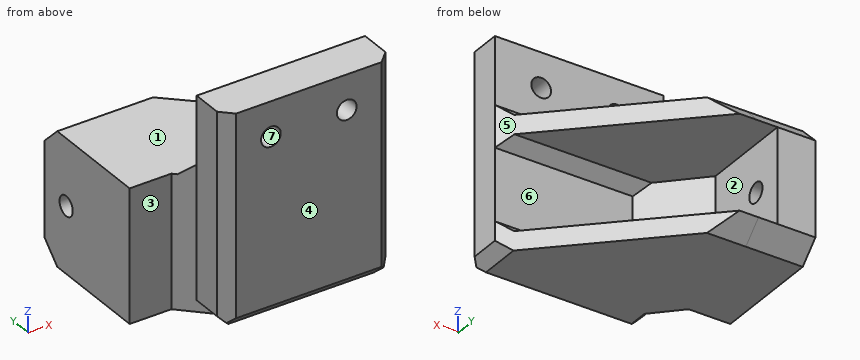
```python
from build123d import *

# Parameters (mm, degrees)
SKETCH2_W                = 44.4
SKETCH2_H                = 55.82
BOSS_EXTRUDE1_DEPTH      = 11
CHAMFER1_SIZE            = 3
SKETCH3_R                = 2.6
CUT_EXTRUDE1_DEPTH       = 62.071371362
SKETCH4_W                = 35
SKETCH4_H                = 37.5
SKETCH4_R                = 2.6
BOSS_EXTRUDE2_DEPTH      = 5
BOSS_EXTRUDE7_DEPTH      = 5
BOSS_EXTRUDE9_DEPTH      = 5
CHAMFER8_SIZE            = 5
BOSS_EXTRUDE11_OUTLINE_W = 35
BOSS_EXTRUDE11_OUTLINE_H = 33.5
BOSS_EXTRUDE11_OUTLINE_R = 2.6
BOSS_EXTRUDE11_DEPTH     = 15
CHAMFER10_SIZE           = 5
SKETCH13_W               = 25
SKETCH13_H               = 34.5
CUT_EXTRUDE2_DEPTH       = 10
BOSS_EXTRUDE12_REACH     = 72.435
BOSS_EXTRUDE13_DEPTH     = 25
CHAMFER11_SIZE           = 3


# Read off the part's stored shape, not the designer's step: Boss-Extrude11
# Some blends are built 0.0001 mm under size
with BuildPart() as part:
    # Sketch2 → Boss-Extrude1 (new body)
    with BuildSketch(Plane(origin=(0, 0, 0), x_dir=(1, 0, 0), z_dir=(0, 1, 0))):
        with Locations((0, 27.91)):
            Rectangle(SKETCH2_W, SKETCH2_H)
    extrude(amount=BOSS_EXTRUDE1_DEPTH)

    # Chamfer1
    chamfer1_edges = [part.edges().sort_by_distance(p)[0] for p in [
        (22.2, 0, -27.91),
        (-22.2, 0, -27.91),
    ]]
    chamfer(chamfer1_edges, length=CHAMFER1_SIZE)

    # Sketch3 → Cut-Extrude1 (cut, through all)
    with BuildSketch(Plane(origin=(0, 11, 0), x_dir=(1, 0, 0), z_dir=(0, 1, 0))):
        with Locations(Location((10, 9.15, 0), (0, 0, 270))):
            Circle(SKETCH3_R)
        with Locations(Location((-10, 9.15, 0), (0, 0, 270))):
            Circle(SKETCH3_R)
    extrude(amount=-CUT_EXTRUDE1_DEPTH, mode=Mode.SUBTRACT)

    # Sketch4 → Boss-Extrude2 (add)
    with BuildSketch(Plane.ZY.offset(22.2)):
        with Locations((-38.32, 29.75)):
            Rectangle(SKETCH4_W, SKETCH4_H)
        with Locations((-38.32, 40)):
            Circle(SKETCH4_R, mode=Mode.SUBTRACT)
    extrude(amount=-BOSS_EXTRUDE2_DEPTH)

    # Sketch8 → Boss-Extrude7 (add)
    with BuildSketch(Plane(origin=(0, 0, -55.82), x_dir=(-1, 0, 0), z_dir=(0, 0, -1))):
        Polygon((-22.2, 11), (22.2, 11), (22.2, 48.5), (17.2, 48.5), align=None)
    extrude(amount=-BOSS_EXTRUDE7_DEPTH)

    # Sketch9 → Boss-Extrude9 (add)
    with BuildSketch(Plane.XY.offset(-20.82)):
        Polygon((-22.2, 11), (-22.2, 48.5), (-17.2, 48.5), (22.2, 11), align=None)
    extrude(amount=-BOSS_EXTRUDE9_DEPTH)

    # Chamfer8
    chamfer8_edges = [part.edges().sort_by_distance(p)[0] for p in [
        (-19.7, 48.5, -20.82),
        (-19.7, 48.5, -55.82),
    ]]
    chamfer(chamfer8_edges, length=CHAMFER8_SIZE)

    # Boss-Extrude11 outline → Boss-Extrude11 (add)
    with BuildSketch(Plane.ZY.offset(22.2)):
        with Locations((-38.32, 31.75)):
            Rectangle(BOSS_EXTRUDE11_OUTLINE_W, BOSS_EXTRUDE11_OUTLINE_H)
        with Locations((-38.32, 40)):
            Circle(BOSS_EXTRUDE11_OUTLINE_R, mode=Mode.SUBTRACT)
    extrude(amount=BOSS_EXTRUDE11_DEPTH)

    # Chamfer10
    chamfer10_edges = [part.edges().sort_by_distance(p)[0] for p in [
        (-29.7, 48.5, -20.82),
        (-29.7, 48.5, -55.82),
    ]]
    chamfer(chamfer10_edges, length=CHAMFER10_SIZE - 0.0001)  # a hair under: the kernel refuses the full size

    # Sketch13 → Cut-Extrude2 (cut)
    with BuildSketch(Plane(origin=(-17.2, 0, 0), x_dir=(0, 0, -1), z_dir=(1, 0, 0))):
        with Locations((38.32, 31.25)):
            Rectangle(SKETCH13_W, SKETCH13_H)
    extrude(amount=-CUT_EXTRUDE2_DEPTH, mode=Mode.SUBTRACT)

    # Boss-Extrude12: up to this face of the body (flat: up to its plane)
    boss_extrude12_end = Plane(part.part.faces().sort_by_distance((-10.417387127, 20.265645238, -55.82))[0])
    # Sketch14 → Boss-Extrude12 (add, up to the picked face)
    with BuildSketch(Plane.XY.offset(-20.82), mode=Mode.PRIVATE) as boss_extrude12_sk1:
        Polygon((-22.2, 15), (-26.2, 15), (-22.2, 11), align=None)
    boss_extrude12_tool1 = split(extrude(boss_extrude12_sk1.sketch, amount=-BOSS_EXTRUDE12_REACH, mode=Mode.PRIVATE), bisect_by=boss_extrude12_end, keep=Keep.BOTH, mode=Mode.PRIVATE)
    add(boss_extrude12_tool1.solids().sort_by(Axis((-23.533333, 13.666667, -20.82), (0, 0, -1)))[0])

    # Sketch15 → Boss-Extrude13 (add)
    with BuildSketch(Plane(origin=(0, 0, -25.82), x_dir=(-1, 0, 0), z_dir=(0, 0, -1))):
        Polygon((14.118524548, 11), (27.2, 24.081475452), (27.2, 15), (22.2, 15), (22.2, 11), align=None)
    extrude(amount=BOSS_EXTRUDE13_DEPTH)

    # Chamfer11
    # the kernel refuses this chamfer: 3 mm, written as the material it adds along each edge
    with BuildSketch(Plane(origin=(22.2, 11, -50.82), x_dir=(0, 0.9996219169112968, -0.027495876610589085), z_dir=(-1, 0, 0))) as chamfer11_piece_1_section:
        Polygon((CHAMFER11_SIZE * 0.999621916911, -CHAMFER11_SIZE * 0.0274958766106), (-CHAMFER11_SIZE * 0.0274958766106, -CHAMFER11_SIZE * 0.999621916911), (0, 0), align=None)
    chamfer11_piece_1 = extrude(amount=44.033573512, mode=Mode.PRIVATE)
    chamfer11_piece_1 = split(chamfer11_piece_1, bisect_by=Plane(origin=(11.645849557, 21.045193949, -49.830255653), z_dir=(-0.689425602489498, -0.7243564996822992, 0)), keep=Keep.TOP, mode=Mode.PRIVATE)
    add(chamfer11_piece_1)
    with BuildSketch(Plane(origin=(22.2, 11, -25.82), x_dir=(0, -0.027495876610589064, -0.9996219169112965), z_dir=(-1, 0, 0))) as chamfer11_piece_2_section:
        Polygon((CHAMFER11_SIZE * 0.999621916911, -CHAMFER11_SIZE * 0.0274958766106), (-CHAMFER11_SIZE * 0.0274958766106, -CHAMFER11_SIZE * 0.999621916911), (0, 0), align=None)
    chamfer11_piece_2 = extrude(amount=44.033573512, mode=Mode.PRIVATE)
    chamfer11_piece_2 = split(chamfer11_piece_2, bisect_by=Plane(origin=(11.645849557, 21.045193949, -26.809744347), z_dir=(-0.6894256024894981, -0.7243564996822992, 0)), keep=Keep.TOP, mode=Mode.PRIVATE)
    add(chamfer11_piece_2)
    with BuildSketch(Plane(origin=(22.2, 11, -20.82), x_dir=(0, 0.9996219169112968, -0.027495876610587933), z_dir=(-1, 0, 0))) as chamfer11_piece_3_section:
        Polygon((CHAMFER11_SIZE * 0.999621916911, -CHAMFER11_SIZE * 0.0274958766106), (-CHAMFER11_SIZE * 0.0274958766106, -CHAMFER11_SIZE * 0.999621916911), (0, 0), align=None)
    chamfer11_piece_3 = extrude(amount=44.4, mode=Mode.PRIVATE)
    chamfer11_piece_3 = split(chamfer11_piece_3, bisect_by=Plane(origin=(9.795664895, 22.806156509, -19.82331844), z_dir=(-0.6894256024894981, -0.7243564996822992, 0)), keep=Keep.TOP, mode=Mode.PRIVATE)
    chamfer11_piece_3 = split(chamfer11_piece_3, bisect_by=Plane(origin=(-11.844103609, 0.644103609, -19.82331844), z_dir=(0.7071067811865474, 0.7071067811865477, 0)), keep=Keep.TOP, mode=Mode.PRIVATE)
    add(chamfer11_piece_3)
    with BuildSketch(Plane(origin=(22.2, 11, -20.82), x_dir=(0, 0.9996219169112968, -0.027495876610587933), z_dir=(-1, 0, 0))) as chamfer11_piece_4_section:
        Polygon((CHAMFER11_SIZE * 0.999621916911, -CHAMFER11_SIZE * 0.0274958766106), (-CHAMFER11_SIZE * 0.0274958766106, -CHAMFER11_SIZE * 0.999621916911), (0, 0), align=None)
    chamfer11_piece_4 = extrude(amount=52.115048964, mode=Mode.PRIVATE)
    chamfer11_piece_4 = split(chamfer11_piece_4, bisect_by=Plane(origin=(-23.372890722, 12.172890722, -20.136626916), z_dir=(0.7071067811865474, 0.7071067811865477, 0)), keep=Keep.TOP, mode=Mode.PRIVATE)
    chamfer11_piece_4 = split(chamfer11_piece_4, bisect_by=Plane(origin=(-22.2, 12.563854296, -20.136626916), z_dir=(-1, 0, 0)), keep=Keep.TOP, mode=Mode.PRIVATE)
    add(chamfer11_piece_4)
    # the kernel refuses this chamfer: 3 mm, written as the material it takes off along each edge
    with BuildSketch(Plane(origin=(-22.2, 18.715048964, -55.82), x_dir=(0.9996219169112965, 0, -0.02749587661058676), z_dir=(0, -1, 0))) as chamfer11_2_piece_1_section:
        Polygon((CHAMFER11_SIZE * 0.999621916911, CHAMFER11_SIZE * 0.0274958766106), (-CHAMFER11_SIZE * 0.0274958766106, CHAMFER11_SIZE * 0.999621916911), (0, 0), align=None)
    chamfer11_2_piece_1 = extrude(amount=23.430097928, mode=Mode.PRIVATE)
    chamfer11_2_piece_1 = split(chamfer11_2_piece_1, bisect_by=Plane(origin=(-17.558310603, 6.358310603, -54.809870411), z_dir=(-0.7071067811865474, -0.7071067811865477, 0)), keep=Keep.TOP, mode=Mode.PRIVATE)
    add(chamfer11_2_piece_1, mode=Mode.SUBTRACT)
    with BuildSketch(Plane(origin=(22.2, -4.715048964, -55.82), x_dir=(-0.9996219169112965, 0, -0.02749587661058676), z_dir=(0, 1, 0))) as chamfer11_2_piece_2:
        Polygon((CHAMFER11_SIZE * 0.999621916911, CHAMFER11_SIZE * 0.0274958766106), (-CHAMFER11_SIZE * 0.0274958766106, CHAMFER11_SIZE * 0.999621916911), (0, 0), align=None)
    extrude(amount=23.430097928, mode=Mode.SUBTRACT)
    with BuildSketch(Plane(origin=(26.915048964, 0, -55.82), x_dir=(0, 0.9996219169112968, -0.027495876610586778), z_dir=(-1, 0, 0))) as chamfer11_2_piece_3:
        Polygon((CHAMFER11_SIZE * 0.999621916911, -CHAMFER11_SIZE * 0.0274958766106), (-CHAMFER11_SIZE * 0.0274958766106, -CHAMFER11_SIZE * 0.999621916911), (0, 0), align=None)
    extrude(amount=53.830097928, mode=Mode.SUBTRACT)


solid = part.part
```
Work out the finished part from the listing and answer in its coordinate system (mm). Face numbers are marked on the shaded views. A direction names the side the tool comes from. Coordinates: 2 decimals unless noted, no trailing zeros. Loops run counter-clockwise (first coordinate to the right, second up) from the corner with the lowest first, then second, coordinate; pieces in that order, holes last.
1) Section D-D (x = 10) is taken. Give the vertices of the cut face in (y, z).
Results:
outline: (0, -52.82) - (3, -55.82) - (22.61, -55.82) - (22.61, -50.82) - (14, -50.82) - (11, -47.82) - (11, -28.82) - (14, -25.82) - (22.61, -25.82) - (22.61, -20.82) - (14, -20.82) - (11, -17.82) - (11, -11.75) - (0, -11.75) - close; (0, -6.55) - (11, -6.55) - (11, 0) - (0, 0) - close
2) Section B-B (x = -28) is taken. Give the vertices of the cut face in (y, z).
Results:
outline: (15, -55.82) - (43.5, -55.82) - (48.5, -50.82) - (48.5, -25.82) - (43.5, -20.82) - (15, -20.82) - close; hole circle Ø5.2 at (40, -38.32)
3) Section A-A (z = -38.32) is taken. Give the vertices of the cut face in (x, y), plus the area to 3 significant figures.
Results:
outline: (-37.2, 15) - (-26.2, 15) - (-22.2, 11) - (-22.2, 3) - (-19.2, 0) - (19.2, 0) - (22.2, 3) - (22.2, 11) - (-14.12, 11) - (-27.2, 24.08) - (-27.2, 37.4) - (-37.2, 37.4) - close; (-37.2, 42.6) - (-27.2, 42.6) - (-27.2, 48.5) - (-37.2, 48.5) - close
area: 836 mm2
4) For a pull along X with two mould halves and no side action, classify the marked faces 5, 6 and 7 as +X half, -X half, draft (parallel to the pull), parting line (faces both ways), or undercut.
Results:
face 5: +X half
face 6: draft
face 7: undercut
5) Flat-ended cylindrical pins translate along their axes: pin 1 (4.5 mm diameter, centred on y = 40, z = -38.32, fed in from +X); pin 2 (8.5 mm diameter, centred on x = -10, z = -9.15, fed in from +Y); pin 3 (10.5 mm diameter, centred on x = -6, y = 31.5, fed in from +Z); pin 4 (5.5 mm diameter, centred on y = 46.5, z = -53, fed in from +X). Find the tip coordinate at first contact, or state that the pin passes through.
Results:
pin 1: passes through
pin 2: stops at y = 11
pin 3: stops at z = -20.82
pin 4: stops at x = -12.21
6) Section C-C (z = -9.15) is taken. Give the vertices of the cut face in (x, y).
Results:
outline: (-22.2, 3) - (-19.2, 0) - (-12.6, 0) - (-12.6, 11) - (-22.2, 11) - close; (-7.4, 0) - (7.4, 0) - (7.4, 11) - (-7.4, 11) - close; (12.6, 0) - (19.2, 0) - (22.2, 3) - (22.2, 11) - (12.6, 11) - close
7) For the marked faces 1, 2, 3 and 4, determine the directions among +Z, -Z, +X, -X, +Y, -Y from which every point of the face is accessible in a straight line to the end or side of a thin tool.
Results:
face 1: +Z, +X, -X, +Y
face 2: +X, +Y
face 3: +Z, -Z, -X, -Y
face 4: +Z, -Z, +X, -X, -Y
8) Consider probe 1 along X at (y, z) = (5.25, -9.15); probe 2 along Z at (x, y) = (-9.5, 19); probe 3 along Z at (x, y) = (-34, 40). Determine where each line is inside the solid, lowest interval first.
Results:
probe 1: x = -22.2 to -12.6, -7.4 to 7.4, 12.6 to 22.2
probe 2: z = -55.82 to -50.82, -25.82 to -20.82
probe 3: z = -55.82 to -40.92, -35.72 to -20.82
